Autodesk Inventor part; units mm, degrees
ref_plane "YZ Plane" through (0, 0, 0) normal (1, 0, 0) x (0, 1, 0)
ref_plane "XZ Plane" through (0, 0, 0) normal (0, 1, 0) x (-1, 0, 0)
ref_plane "XY Plane" through (0, 0, 0) normal (0, 0, 1) x (1, 0, 0)
sketch "Sketch1" plane through (0, 0, 0) normal (0, 0, 1) x (1, 0, 0)
  line L0 (0, 0) -> (124, 0)
  line L1 (124, 0) -> (124, 129)
  line L2 (124, 129) -> (0, 129)
  line L3 (0, 129) -> (0, 0)
  circle A0 centre (62, 19.5) radius 2.5
  point P0 (62, 0)
  dimension "d0" = 124
  dimension "d1" = 129
  dimension "d2" = 5
  dimension "d3" = 19.5
extrude "Extrusion1" add sketch "Sketch1" along normal blind 10
sketch "Sketch2" plane through (0, 0, 10) normal (0, 0, 1) x (1, 0, 0)
  line L0 (0, 82) -> (-10, 82)
  line L1 (-10, 82) -> (-10, 42)
  line L2 (-10, 42) -> (0, 42)
  line L3 (0, 42) -> (0, 82)
  circle A0 centre (-5, 62) radius 2.5
  line L4 (0, 124) -> (0, 0)
  line L5 (0, 129) -> (0, 0)
  point P0 (-10, 62)
  point P1 (0, 62)
  point P2 (-5, 82)
  point P3 (0, 62)
  dimension "d8" = 10
  dimension "d9" = 40
  dimension "d10" = 5
  dimension "d27" = 124
extrude "Extrusion2" add sketch "Sketch2" against normal blind 5
sketch "Sketch3" plane through (0, 0, 10) normal (0, 0, 1) x (1, 0, 0)
  line L0 (124, 41) -> (112, 41)
  line L1 (112, 41) -> (112, 83)
  line L2 (112, 83) -> (124, 83)
  line L3 (124, 83) -> (124, 41)
  line L4 (124, 0) -> (124, 129)
  line L5 (124, 124) -> (124, 0)
  point P0 (0, 0)
  point P1 (112, 62)
  point P2 (124, 62)
  point P3 (124, 62)
  dimension "d13" = 12
  dimension "d14" = 42
  dimension "d28" = 124
extrude "Extrusion3" cut sketch "Sketch3" against normal blind 6
sketch "Sketch4" plane through (0, 0, 4) normal (0, 0, 1) x (1, 0, 0)
  line L0 (124, 41) -> (112, 41) construction
  line L1 (124, 83) -> (124, 41) construction
  line L2 (112, 83) -> (124, 83) construction
  line L3 (112, 41) -> (112, 83) construction
  circle A0 centre (119, 62) radius 2.5
  point P0 (0, 0)
  point P1 (124, 62)
  point P2 (118, 41)
  dimension "d17" = 5
  dimension "d29" = 5
extrude "Extrusion4" cut sketch "Sketch4" against normal through all
properties part number "TA002" material "ABS Plastic"
Part model, mm, in its own coordinate system. A direction names the side the tool comes from. Round coordinates to 2 decimals unless told otherwise and drop trailing zeros. Order: outer loops, then holes, each group sorted by start corner. A loop starts at its lowest first (then second) coordinate and runs counter-clockwise, first axis right, second up. Notation, with made-up numbers: (53, -11.5) -> (111, -11.5) arc R20 cw to (111, 5.5) -> close; hole circle Ø9 at (24.5, 69.25). An arc over 180 degrees is marked (long way). Put each result on its own line as item: value.
Q1. Band-saw the part on C-C (z = 7.75). Give the cut face in (x, y), and give its area (3 significant figures).
From the geometry:
outline: (-10, 42) -> (0, 42) -> (0, 0) -> (124, 0) -> (124, 41) -> (112, 41) -> (112, 83) -> (124, 83) -> (124, 129) -> (0, 129) -> (0, 82) -> (-10, 82) -> close; hole circle Ø5 at (-5, 62); hole circle Ø5 at (62, 19.5)
area: 15,900 mm2
Q2. Band-saw the part on D-D (y = 19.5). Give the cut face in (x, z).
From the geometry:
outline: (0, 0) -> (59.5, 0) -> (59.5, 10) -> (0, 10) -> close; (64.5, 0) -> (124, 0) -> (124, 10) -> (64.5, 10) -> close
Q3. Wall check: line 1 (Y direction, x = 119, z = 1.4); line 2 (Y direction, x = 116, z = 7.75); line 3 (X direction, y = 90, z = 3). Give the ranges that are in metal, low to high. Write a range as [from, to].
From the geometry:
line 1: y = [0, 59.5], [64.5, 129]
line 2: y = [0, 41], [83, 129]
line 3: x = [0, 124]
Q4. Pin check, flat tips, straight feed: pin 1 Ø6.5 at (x, y) = (119, 62) entering from -Z; pin 2 Ø5.5 at (x, z) = (-5.5, 7.5) entering from -Y; pin 3 Ø5.5 at (x, z) = (-4.5, 8) entering from +Y; pin 4 Ø3.5 at (x, y) = (120.5, 63) entering from +Z. Stop position of each tip, or through.
From the geometry:
pin 1: stops at z = 0
pin 2: stops at y = 42
pin 3: stops at y = 82
pin 4: stops at z = 4
Q5. Tool access for faces 4 (the face through (118, 83, 7)), 5 (the face through (-5, 82, 8)), 6 (the face through (-5, 42, 8)), 7 (the face through (121.385, 62.751, 2.028)): list every direction of +Z, -Z, +X, -X, +Y, -Y with a clear straight run to the whole face (end or side of a thin tool).
From the geometry:
face 4: +Z, +X
face 5: +Z, -Z, -X, +Y
face 6: +Z, -Z, -X, -Y
face 7: +Z, -Z
Q6. Pull direction Y, two halves, no side cores. Call faces 1 (the face through (-2.615, 62.751, 7.535)), 2 (the face through (-8, 62, 5)), 3 (the face through (63, 129, 5)): pulls with the +Y half, pulls with the -Y half, needs draft (parallel to the pull), parting line crosses it, or undercut.
From the geometry:
face 1: undercut
face 2: needs draft
face 3: pulls with the +Y half
Q7. Band-saw the part on A-A (x = -5). Give the cut face in (y, z).
From the geometry:
outline: (42, 5) -> (59.5, 5) -> (59.5, 10) -> (42, 10) -> close; (64.5, 5) -> (82, 5) -> (82, 10) -> (64.5, 10) -> close
Q8. Band-saw the part on B-B (y = 62). Give the cut face in (x, z), and give its area (3 significant figures).
From the geometry:
outline: (-10, 5) -> (-7.5, 5) -> (-7.5, 10) -> (-10, 10) -> close; (-2.5, 5) -> (0, 5) -> (0, 0) -> (116.5, 0) -> (116.5, 4) -> (112, 4) -> (112, 10) -> (-2.5, 10) -> close; (121.5, 0) -> (124, 0) -> (124, 4) -> (121.5, 4) -> close
area: 1,170 mm2
